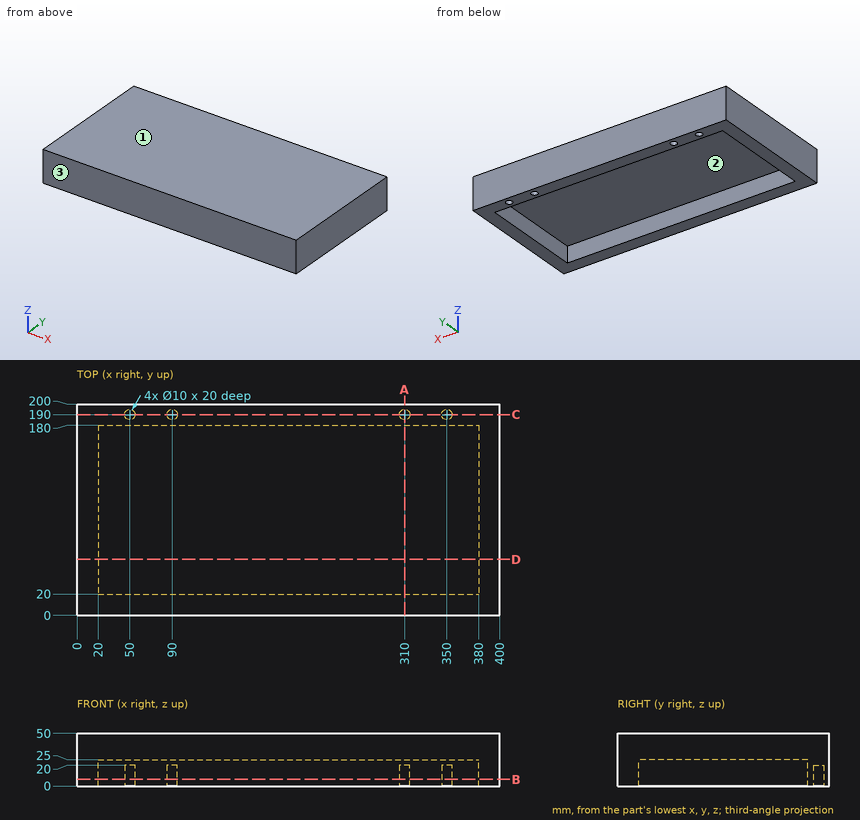
Input: dimensioned drawing with shaded views. Units: mm. Origin: part minimum x, y, z. Coordinates: 2 decimals unless noted, no trailing zeros. Write each loop counter-clockwise with the first axis right and the second up, starting at its lowest first coordinate (ties: lowest second). Pieces come first, ordered by that corner, then holes. Notation, with made-up numbers: M 18,55 L 72,55 A22 cw 72,67 Z; hole C 0.25,83 d5. An arc over 180 degrees is marked long. Answer as a JSON object with one key per item and string values. Group by question number.
(1) Contact query for flat-ended pins moving along their axis: P1, Ø2, axis at x = 121, y = 104, coming from the -Z side; P2, Ø5, axis at x = 92, y = 189, coming from the -Z side. Output: stop coordinate, or through.
(2) Section D-D on y = 53. Output: boundary loops of the cut face in (x, z), plus the area to 3 significant figures.
(3) Ray query, line 1 along Y through (x, z) = (310, 15); line 2 along X through (y, z) = (190, 12.75); line 3 along X through (y, z) = (172.5, 11). Return the intervals inside material, ascending. Write a range as [from, to].
(4) Section B-B on z = 6.5. Output: boundary loops of the cut face in (x, y).
(5) Mould query, pull axis Y, two halves, no side actions, for the marked faces 1, 2 and 3. Classes: pulls with the +Y half, pulls with the -Y half, needs draft (parallel to the pull), parting line crosses it, or undercut.
(6) Section A-A on x = 310. Output: boundary loops of the cut face in (y, z).
(7) Section C-C on y = 190. Output: boundary loops of the cut face in (x, z), plus the area to 3 significant figures.
Result set:
{
 "1": {"P1": "stops at z = 25", "P2": "stops at z = 20"},
 "2": {"outline": "M 0,0 L 20,0 L 20,25 L 380,25 L 380,0 L 400,0 L 400,50 L 0,50 Z", "area": "11,000 mm2"},
 "3": {"line 1": "y = [0, 20], [180, 185], [195, 200]", "line 2": "x = [0, 45], [55, 85], [95, 305], [315, 345], [355, 400]", "line 3": "x = [0, 20], [380, 400]"},
 "4": {"outline": "M 0,0 L 400,0 L 400,200 L 0,200 Z; hole M 20,20 L 380,20 L 380,180 L 20,180 Z; hole C 50,190 d10; hole C 90,190 d10; hole C 310,190 d10; hole C 350,190 d10"},
 "5": {"face 1": "needs draft", "face 2": "undercut", "face 3": "pulls with the -Y half"},
 "6": {"outline": "M 0,0 L 20,0 L 20,25 L 180,25 L 180,0 L 185,0 L 185,20 L 195,20 L 195,0 L 200,0 L 200,50 L 0,50 Z"},
 "7": {"outline": "M 0,0 L 45,0 L 45,20 L 55,20 L 55,0 L 85,0 L 85,20 L 95,20 L 95,0 L 305,0 L 305,20 L 315,20 L 315,0 L 345,0 L 345,20 L 355,20 L 355,0 L 400,0 L 400,50 L 0,50 Z", "area": "19,200 mm2"}
}
